```python
from build123d import *

# Parameters (mm, degrees)
EXTRUDE_1_DEPTH     = 7.8
SKETCH_2_R          = 7
EXTRUDE_2_DEPTH     = 1.2
SKETCH_3_R          = 7
EXTRUDE_3_DEPTH     = 7
SKETCH_4_R          = 2.5
CUT_EXTRUDE_1_DEPTH = 17
SKETCH_6_R          = 2
CUT_EXTRUDE_2_DEPTH = 8
SKETCH_7_R          = 2
CUT_EXTRUDE_3_DEPTH = 8.0000001


with BuildPart() as part:
    # 草图1 → 凸台-拉伸1 (new body)
    with BuildSketch(Plane.XY):
        with BuildLine():
            Line((4.999238476, -0.087262032), (5.941608412, -0.835038606))
            ThreePointArc((5.941608412, -0.835038606), (5.926130044, -0.93860679), (5.908846518, -1.041889066))
            Line((5.908846518, -1.041889066), (4.78152378, -1.461858524))
            ThreePointArc((4.78152378, -1.461858524), (4.755282581, -1.545084972), (4.727592878, -1.627840772))
            Line((4.727592878, -1.627840772), (5.392764278, -2.630226881))
            ThreePointArc((5.392764278, -2.630226881), (5.346039145, -2.723942998), (5.297685557, -2.816829377))
            Line((5.297685557, -2.816829377), (4.095760221, -2.867882182))
            ThreePointArc((4.095760221, -2.867882182), (4.045084972, -2.938926261), (3.99317755, -3.009075116))
            Line((3.99317755, -3.009075116), (4.316038802, -4.167950223))
            ThreePointArc((4.316038802, -4.167950223), (4.242640687, -4.242640687), (4.167950223, -4.316038802))
            Line((4.167950223, -4.316038802), (3.009075116, -3.99317755))
            ThreePointArc((3.009075116, -3.99317755), (2.938926261, -4.045084972), (2.867882182, -4.095760221))
            Line((2.867882182, -4.095760221), (2.816829377, -5.297685557))
            ThreePointArc((2.816829377, -5.297685557), (2.723942998, -5.346039145), (2.630226881, -5.392764278))
            Line((2.630226881, -5.392764278), (1.627840772, -4.727592878))
            ThreePointArc((1.627840772, -4.727592878), (1.545084972, -4.755282581), (1.461858524, -4.78152378))
            Line((1.461858524, -4.78152378), (1.041889066, -5.908846518))
            ThreePointArc((1.041889066, -5.908846518), (0.93860679, -5.926130044), (0.835038606, -5.941608412))
            Line((0.835038606, -5.941608412), (0.087262032, -4.999238476))
            ThreePointArc((0.087262032, -4.999238476), (0, -5), (-0.087262032, -4.999238476))
            Line((-0.087262032, -4.999238476), (-0.835038606, -5.941608412))
            ThreePointArc((-0.835038606, -5.941608412), (-0.93860679, -5.926130044), (-1.041889066, -5.908846518))
            Line((-1.041889066, -5.908846518), (-1.461858524, -4.78152378))
            ThreePointArc((-1.461858524, -4.78152378), (-1.545084972, -4.755282581), (-1.627840772, -4.727592878))
            Line((-1.627840772, -4.727592878), (-2.630226881, -5.392764278))
            ThreePointArc((-2.630226881, -5.392764278), (-2.723942998, -5.346039145), (-2.816829377, -5.297685557))
            Line((-2.816829377, -5.297685557), (-2.867882182, -4.095760221))
            ThreePointArc((-2.867882182, -4.095760221), (-2.938926261, -4.045084972), (-3.009075116, -3.99317755))
            Line((-3.009075116, -3.99317755), (-4.167950223, -4.316038802))
            ThreePointArc((-4.167950223, -4.316038802), (-4.242640687, -4.242640687), (-4.316038802, -4.167950223))
            Line((-4.316038802, -4.167950223), (-3.99317755, -3.009075116))
            ThreePointArc((-3.99317755, -3.009075116), (-4.045084972, -2.938926261), (-4.095760221, -2.867882182))
            Line((-4.095760221, -2.867882182), (-5.297685557, -2.816829377))
            ThreePointArc((-5.297685557, -2.816829377), (-5.346039145, -2.723942998), (-5.392764278, -2.630226881))
            Line((-5.392764278, -2.630226881), (-4.727592878, -1.627840772))
            ThreePointArc((-4.727592878, -1.627840772), (-4.755282581, -1.545084972), (-4.78152378, -1.461858524))
            Line((-4.78152378, -1.461858524), (-5.908846518, -1.041889066))
            ThreePointArc((-5.908846518, -1.041889066), (-5.926130044, -0.93860679), (-5.941608412, -0.835038606))
            Line((-5.941608412, -0.835038606), (-4.999238476, -0.087262032))
            ThreePointArc((-4.999238476, -0.087262032), (-5, 0), (-4.999238476, 0.087262032))
            Line((-4.999238476, 0.087262032), (-5.941608412, 0.835038606))
            ThreePointArc((-5.941608412, 0.835038606), (-5.926130044, 0.93860679), (-5.908846518, 1.041889066))
            Line((-5.908846518, 1.041889066), (-4.78152378, 1.461858524))
            ThreePointArc((-4.78152378, 1.461858524), (-4.755282581, 1.545084972), (-4.727592878, 1.627840772))
            Line((-4.727592878, 1.627840772), (-5.392764278, 2.630226881))
            ThreePointArc((-5.392764278, 2.630226881), (-5.346039145, 2.723942998), (-5.297685557, 2.816829377))
            Line((-5.297685557, 2.816829377), (-4.095760221, 2.867882182))
            ThreePointArc((-4.095760221, 2.867882182), (-4.045084972, 2.938926261), (-3.99317755, 3.009075116))
            Line((-3.99317755, 3.009075116), (-4.316038802, 4.167950223))
            ThreePointArc((-4.316038802, 4.167950223), (-4.242640687, 4.242640687), (-4.167950223, 4.316038802))
            Line((-4.167950223, 4.316038802), (-3.009075116, 3.99317755))
            ThreePointArc((-3.009075116, 3.99317755), (-2.938926261, 4.045084972), (-2.867882182, 4.095760221))
            Line((-2.867882182, 4.095760221), (-2.816829377, 5.297685557))
            ThreePointArc((-2.816829377, 5.297685557), (-2.723942998, 5.346039145), (-2.630226881, 5.392764278))
            Line((-2.630226881, 5.392764278), (-1.627840772, 4.727592878))
            ThreePointArc((-1.627840772, 4.727592878), (-1.545084972, 4.755282581), (-1.461858524, 4.78152378))
            Line((-1.461858524, 4.78152378), (-1.041889066, 5.908846518))
            ThreePointArc((-1.041889066, 5.908846518), (-0.93860679, 5.926130044), (-0.835038606, 5.941608412))
            Line((-0.835038606, 5.941608412), (-0.087262032, 4.999238476))
            ThreePointArc((-0.087262032, 4.999238476), (0, 5), (0.087262032, 4.999238476))
            Line((0.087262032, 4.999238476), (0.835038606, 5.941608412))
            ThreePointArc((0.835038606, 5.941608412), (0.93860679, 5.926130044), (1.041889066, 5.908846518))
            Line((1.041889066, 5.908846518), (1.461858524, 4.78152378))
            ThreePointArc((1.461858524, 4.78152378), (1.545084972, 4.755282581), (1.627840772, 4.727592878))
            Line((1.627840772, 4.727592878), (2.630226881, 5.392764278))
            ThreePointArc((2.630226881, 5.392764278), (2.723942998, 5.346039145), (2.816829377, 5.297685557))
            Line((2.816829377, 5.297685557), (2.867882182, 4.095760221))
            ThreePointArc((2.867882182, 4.095760221), (2.938926261, 4.045084972), (3.009075116, 3.99317755))
            Line((3.009075116, 3.99317755), (4.167950223, 4.316038802))
            ThreePointArc((4.167950223, 4.316038802), (4.242640687, 4.242640687), (4.316038802, 4.167950223))
            Line((4.316038802, 4.167950223), (3.99317755, 3.009075116))
            ThreePointArc((3.99317755, 3.009075116), (4.045084972, 2.938926261), (4.095760221, 2.867882182))
            Line((4.095760221, 2.867882182), (5.297685557, 2.816829377))
            ThreePointArc((5.297685557, 2.816829377), (5.346039145, 2.723942998), (5.392764278, 2.630226881))
            Line((5.392764278, 2.630226881), (4.727592878, 1.627840772))
            ThreePointArc((4.727592878, 1.627840772), (4.755282581, 1.545084972), (4.78152378, 1.461858524))
            Line((4.78152378, 1.461858524), (5.908846518, 1.041889066))
            ThreePointArc((5.908846518, 1.041889066), (5.926130044, 0.93860679), (5.941608412, 0.835038606))
            Line((5.941608412, 0.835038606), (4.999238476, 0.087262032))
            ThreePointArc((4.999238476, 0.087262032), (5, 0), (4.999238476, -0.087262032))
        make_face()
    extrude(amount=EXTRUDE_1_DEPTH)

    # 草图2 → 凸台-拉伸2 (add)
    with BuildSketch(Plane.XY.offset(7.8)):
        Circle(SKETCH_2_R)
    extrude(amount=EXTRUDE_2_DEPTH)

    # 草图3 → 凸台-拉伸3 (add)
    with BuildSketch(Plane(origin=(0, 0, 0), x_dir=(-1, 0, 0), z_dir=(0, 0, -1))):
        Circle(SKETCH_3_R)
    extrude(amount=EXTRUDE_3_DEPTH)

    # 草图4 → 切除-拉伸1 (cut, through all)
    with BuildSketch(Plane(origin=(0, 0, -7), x_dir=(-1, 0, 0), z_dir=(0, 0, -1))):
        Circle(SKETCH_4_R)
    extrude(amount=-CUT_EXTRUDE_1_DEPTH, mode=Mode.SUBTRACT)

    # 草图6 → 切除-拉伸2 (cut, through all)
    with BuildSketch(Plane(origin=(0, 0, 0), x_dir=(1, 0, 0), z_dir=(0, 1, 0))):
        with Locations((0, 3.5)):
            Circle(SKETCH_6_R)
    extrude(amount=-CUT_EXTRUDE_2_DEPTH, mode=Mode.SUBTRACT)

    # 草图7 → 切除-拉伸3 (cut, through all)
    with BuildSketch(Plane(origin=(0, 0, 0), x_dir=(0, 0, -1), z_dir=(1, 0, 0))):
        with Locations((3.5, 0)):
            Circle(SKETCH_7_R)
    extrude(amount=-CUT_EXTRUDE_3_DEPTH, mode=Mode.SUBTRACT)


solid = part.part
```
Build history of the part. All positions in model axes, mm. A direction names the side the tool comes from. Give positions to 0.01 mm unless a question says otherwise; leave off trailing zeros. Order: outer loops, then holes, each group sorted by start corner. A loop starts at its lowest first (then second) coordinate and runs counter-clockwise, first axis right, second up. Notation, with made-up numbers: M 9.5,78 L 15.5,78 A25 cw 15.5,99 Z; hole C 32,88 d6. An arc over 180 degrees is marked long. Write item = value, one per line. Start each with the question number.
(1) Probe L1, parallel to Z at x = -5.7, y = 0; L2, parallel to Z at x = -3.2, y = 0; L3, parallel to Z at x = 1.75, y = 5.5. List the from-to ranges inside material, lowest first. Write a range as [from, to].
(2) Pin check, flat tips, straight feed: pin 1 Ø4 at (x, z) = (3, 3.5) entering from +Y; pin 2 Ø6 at (y, z) = (-4.5, 0.5) entering from +X; pin 3 Ø5 at (y, z) = (4.5, -2.5) entering from -X. Stop position of each tip, or through.
(3) Slice it at D-D on y = 3.75. Write the cut outline in (x, z), plus the area to 3 significant figures.
(4) Slice it at B-B on z = -3.5. Write the cut outline in (x, y), plus the area to 3 significant figures.
(5) Slice it at A-A on x = -1.25. Write the cut outline in (y, z), plus the area to 3 significant figures.
(6) Slice it at C-C on y = -2.25. Write the cut outline in (x, z), plus the area to 3 significant figures.
(7) Two-plate mould, pull along Y, no slides. Class faces 1 (the flat face through (2.843, -4.688, 3.845)), 2 (the cylindrical face through (-4.823, 1.352, -2.026)), 3 (the flat face through (0, -3, 9)), 4 (the flat face through (5.065, 2.136, 3.845)): released by +Y, released by -Y, zero draft, split by the parting line, or undercut.
(8) Which spindle directions (+Z, -Z, +X, -X, +Y, -Y) get a long thin tool onto all of the face, cutting with end or side? Do faces 5 (the flat face through (5.056, -2.122, 3.845)), 6 (the flat face through (-3.58, -4.152, 3.845)), 7 (the flat face through (3, -5, 7.8)), 8 (the flat face through (-5.464, 0.456, 3.845)), 9 (the flat face through (-3.597, 4.157, 3.845)). Say none if no direction does.
Responses:
q1.L1 = [-7, -5.5], [-1.5, 0], [7.8, 9]
q1.L2 = [-7, -5.5], [-1.5, 9]
q1.L3 = [-7, 0], [7.8, 9]
q2.pin_1 = 5.92
q2.pin_2 = 6.83
q2.pin_3 = -6.71
q3.outline = M -5.91,-7 L 5.91,-7 L 5.91,0 L 4.2,0 L 4.2,7.8 L 5.91,7.8 L 5.91,9 L -5.91,9 L -5.91,7.8 L -4.2,7.8 L -4.2,0 L -5.91,0 Z
q3.area = 162 mm2
q4.outline = M -6.71,-2 A7 ccw -2,-6.71 L -2,-2 Z; M -6.71,2 L -1.5,2 A2.5 cw 2,-1.5 L 2,-6.71 A7 ccw long Z
q4.area = 96.8 mm2
q5.outline = M -6.89,-7 L -2.17,-7 L -2.17,-5.06 L -6.89,-5.06 Z; M -6.89,-1.94 L -2.17,-1.94 L -2.17,9 L -6.89,9 L -6.89,7.8 L -5.35,7.8 L -5.35,0 L -6.89,0 Z; M 2.17,-7 L 6.89,-7 L 6.89,0 L 5.35,0 L 5.35,7.8 L 6.89,7.8 L 6.89,9 L 2.17,9 Z
q5.area = 112 mm2
q6.outline = M -6.63,-7 L -1.09,-7 L -1.09,-5.18 A2 cw -1.09,-1.82 L -1.09,9 L -6.63,9 L -6.63,7.8 L -5.14,7.8 L -5.14,0 L -6.63,0 Z; M 1.09,-7 L 6.63,-7 L 6.63,0 L 5.14,0 L 5.14,7.8 L 6.63,7.8 L 6.63,9 L 1.09,9 L 1.09,-1.82 A2 cw 1.09,-5.18 Z
q6.area = 150 mm2
q7.face_1 = released by -Y
q7.face_2 = undercut
q7.face_3 = zero draft
q7.face_4 = undercut
q8.face_5 = +X
q8.face_6 = -Y
q8.face_7 = none
q8.face_8 = -X
q8.face_9 = +Y
